```python
from build123d import *

# Parameters (mm, degrees)
SKETCH_1_W          = 17
SKETCH_1_H          = 16
SKETCH_1_R          = 1
SKETCH_1_R_2        = 4
EXTRUDE_1_DEPTH     = 4
EXTRUDE_2_DEPTH     = 16
SKETCH_4_R          = 1
CUT_EXTRUDE_1_DEPTH = 16
FILLET_1_R          = 2
FILLET_2_R          = 5
SKETCH_7_W          = 6
SKETCH_7_H          = 80
CUT_EXTRUDE_2_DEPTH = 10
FILLET_3_R          = 1
FILLET_4_R          = 2.5


with BuildPart() as part:
    # 草图1 → 凸台-拉伸1 (new body)
    with BuildSketch(Plane(origin=(0, 0, 0), x_dir=(1, 0, 0), z_dir=(0, 1, 0))):
        Rectangle(SKETCH_1_W, SKETCH_1_H)
        with Locations(Location((6, 4, 0), (0, 0, 270))):
            Circle(SKETCH_1_R, mode=Mode.SUBTRACT)
        with Locations(Location((-6, 4, 0), (0, 0, 90))):
            Circle(SKETCH_1_R, mode=Mode.SUBTRACT)
        with Locations(Location((6, -4, 0), (0, 0, 90))):
            Circle(SKETCH_1_R, mode=Mode.SUBTRACT)
        with Locations(Location((-6, -4, 0), (0, 0, 270))):
            Circle(SKETCH_1_R, mode=Mode.SUBTRACT)
        with Locations(Location((0, 0, 0), (0, 0, 270))):
            Circle(SKETCH_1_R_2, mode=Mode.SUBTRACT)
    extrude(amount=EXTRUDE_1_DEPTH)

    # 草图2 → 凸台-拉伸2 (add)
    with BuildSketch(Plane.XY.offset(8)):
        Polygon((8.5, 4.825938125), (8.5, 0), (13.5, 0), (13.5, 22), (-47.839490213, 79.2), (-50.691220222, 79.2), (-70.881411302, 79.2), (-70.881411302, 75.2), (-51, 75.2), (-50.881411302, 75.2), (8.5, 19.825938125), align=None)
    extrude(amount=-EXTRUDE_2_DEPTH)

    # 草图4 → 切除-拉伸1 (cut)
    with BuildSketch(Plane.XZ.offset(-75.2)):
        with Locations(Location((-54, 4, 0), (0, 0, 270))):
            Circle(SKETCH_4_R)
        with Locations(Location((-54, -4, 0), (0, 0, 270))):
            Circle(SKETCH_4_R)
        with Locations(Location((-66, -4, 0), (0, 0, 270))):
            Circle(SKETCH_4_R)
        with Locations(Location((-66, 4, 0), (0, 0, 270))):
            Circle(SKETCH_4_R)
    extrude(amount=-CUT_EXTRUDE_1_DEPTH, mode=Mode.SUBTRACT)

    # 圆角1
    fillet_1_edges = [part.edges().sort_by_distance(p)[0] for p in [
        (-70.881411302, 77.2, -8),
        (-70.881411302, 77.2, 8),
        (-8.5, 2, 8),
        (-8.5, 2, -8),
    ]]
    fillet(fillet_1_edges, radius=FILLET_1_R)

    # 圆角2
    fillet_2_edges = [part.edges().sort_by_distance(p)[0] for p in [
        (8.5, 19.825938125, 0),
        (-47.839490213, 79.2, 0),
        (13.5, 22, 0),
    ]]
    fillet(fillet_2_edges, radius=FILLET_2_R)

    # 草图7 → 切除-拉伸2 (cut)
    with BuildSketch(Plane(origin=(17.252348355, 18.50087855, 0), x_dir=(0, 0, -1), z_dir=(0.6819983600624965, 0.7313537016191725, 0))):
        with Locations((5, 49.853652648)):
            Rectangle(SKETCH_7_W, SKETCH_7_H)
    extrude(amount=-CUT_EXTRUDE_2_DEPTH, mode=Mode.SUBTRACT)

    # 圆角3
    # the kernel refuses this fillet: 1 mm, written as the material it takes off along each edge
    with BuildSketch(Plane(origin=(-49.057187154, 79.143148127, -2), x_dir=(-0.9996800282081353, 0.02529508256127706, 0), z_dir=(0, 0, -1))) as fillet_3_piece_1:
        with BuildLine():
            CenterArc((2.222251386, -0.999680028), FILLET_3_R, 88.550543928, 133)
            Line((1.473880493, -1.662960516), (1.399043403, -1.729288565))
            Line((1.399043403, -1.729288565), (-0.074837089, -0.066328049))
            Line((-0.074837089, -0.066328049), (-0.012531551, 0.099211694))
            ThreePointArc((-0.012531551, 0.099211694), (0.755582446, 0.13778344), (2.250075977, 0.099968003))
            Line((2.250075977, 0.099968003), (2.247546469, 0))
        make_face()
    extrude(amount=11.618866172, mode=Mode.SUBTRACT)

    # 圆角4
    fillet_4_edges = [part.edges().sort_by_distance(p)[0] for p in [
        (8.340847116, 23.392669243, -2),
        (8.340847116, 23.392669243, -8),
    ]]
    fillet(fillet_4_edges, radius=FILLET_4_R)


solid = part.part
```
Verification items for the finished model (mm, model axes). A direction names the side the tool comes from. Give positions to 0.01 mm unless a question says otherwise; leave off trailing zeros. Loops run counter-clockwise (first coordinate to the right, second up) from the corner with the lowest first, then second, coordinate; pieces in that order, holes last. Notation, with made-up numbers: M -31,40.5 L 14,40.5 A24 cw 14,64.5 Z; hole C 89,23 d3. An arc over 180 degrees is marked long. Return JSON: item names as keys, results as strings.
1) Tool access check on faces 4 (the flat face through (-8.5, 2, 0)), 5 (the flat face through (-51.638, 76.375, -4.958)), 6 (the cylindrical face through (8.097, 19.619, -0.112)). Record the directions out of +Z, -Z, +X, -X, +Y, -Y that give a thin tool (end or side, any length) a straight path to the whole face; none if there is none.
Findings:
{"face 4": "+Z, -Z, -X, -Y", "face 5": "-Z, +X, -Y", "face 6": "+Z, -Z, -X"}
2) Gauge pin test, flat ends, axial feed: P1, Ø7, axis at x = 0, z = 0, coming from the -Y side; P2, Ø2.5, axis at x = 6, z = -4, coming from the +Y side; P3, Ø1.2, axis at x = -54, z = 4, coming from the -Y side; P4, Ø5, axis at x = -60.5, z = 0, coming from the -Y side. Record the tip position at first contact, or that the pin passes through.
Findings:
{"P1": "stops at y = 24.49", "P2": "stops at y = 22.45", "P3": "passes through", "P4": "stops at y = 75.2"}
3) Section check D-D, the plane x = 0. Enter the section's corners in (y, z), and give its area (3 significant figures).
Findings:
{"outline": "M 0,-8 L 4,-8 L 4,-4 L 0,-4 Z; M 0,4 L 4,4 L 4,8 L 0,8 Z; M 27.75,-2 L 34.59,-2 L 34.59,8 L 27.75,8 Z", "area": "100 mm2"}
4) Section check A-A, the plane z = 0. Enter the section's corners in (x, y).
Findings:
{"outline": "M -70.88,75.2 L -50.88,75.2 L 6.91,21.31 A5 cw 8.5,17.65 L 8.5,4 L 4,4 L 4,0 L 13.5,0 L 13.5,19.83 A5 ccw 11.91,23.48 L -46.4,77.86 A5 ccw -49.81,79.2 L -70.88,79.2 Z; M -8.5,0 L -4,0 L -4,4 L -8.5,4 Z"}
5) Section check C-C, the plane y = 15. Enter the section's corners in (x, z), and give its area (3 significant figures).
Findings:
{"outline": "M 8.5,-8 L 13.5,-8 L 13.5,8 L 8.5,8 Z", "area": "80.0 mm2"}
6) Section check B-B, the plane x = -66. Enter the section's corners in (y, z).
Findings:
{"outline": "M 75.2,-8 L 79.2,-8 L 79.2,-5 L 75.2,-5 Z; M 75.2,-3 L 79.2,-3 L 79.2,3 L 75.2,3 Z; M 75.2,5 L 79.2,5 L 79.2,8 L 75.2,8 Z"}
7) Mould release check, pull along Z, two halves, no side actions. Record for faces 1 (the flat face through (-22, 52, -2)), 2 (the cylindrical face through (-6.676, 1.972, -3.263)), 3 (the cylindrical face through (-47.95, 78.84, 2.93)): released by +Z, released by -Z, zero draft, split by the parting line, or undercut.
Findings:
{"face 1": "released by -Z", "face 2": "undercut", "face 3": "zero draft"}
8) Material ranges on L1, parallel to Z at x = -66, y = 77.4; L2, parallel to X at y = 76.7, z = 4; L3, parallel to X at y = 15.5, z = 5.5, recorded low to high. Write a range as [from, to].
Findings:
{"L1": "z = [-8, -5], [-3, 3], [5, 8]", "L2": "x = [-70.88, -67], [-65, -55], [-53, -45.16]", "L3": "x = [8.5, 13.5]"}
